Build history of the part. All positions in model axes, mm. A direction names the side the tool comes from. Give positions to 0.01 mm unless a question says otherwise; leave off trailing zeros. Loops run counter-clockwise (first coordinate to the right, second up) from the corner with the lowest first, then second, coordinate; pieces in that order, holes last. Notation, with made-up numbers: (9, -39.5) -> (61, -39.5) arc R18 cw to (61, -20.5) -> close; hole circle Ø11 at (66.25, 3.25). An arc over 180 degrees is marked (long way). Answer as a JSON object with one key per item and string values. Group by question number.
from build123d import *
from build123d.topology import SkipClean

# Parameters (mm, degrees)
SKETCH1_W           = 54
SKETCH1_H           = 28.5
SKETCH1_W_2         = 5
SKETCH1_H_2         = 22.5
SKETCH1_R           = 1.7
SKETCH1_R_2         = 7.5
BOSS_EXTRUDE2_DEPTH = 3
SKETCH2_W           = 4
SKETCH2_H           = 20.5
BOSS_EXTRUDE3_DEPTH = 21.75
SKETCH4_R           = 10.25
BOSS_EXTRUDE4_DEPTH = 4
SKETCH6_R           = 4.4
SKETCH6_R_2         = 1.45
CUT_EXTRUDE3_DEPTH  = 4
SKETCH7_R           = 1.45
CUT_EXTRUDE4_DEPTH  = 1.5
SKETCH8_W           = 28.781481152
SKETCH8_H           = 28.5
BOSS_EXTRUDE5_DEPTH = 3
SKETCH9_R           = 1.7
CUT_EXTRUDE5_DEPTH  = 3
SKETCH10_W          = 54
SKETCH10_H          = 28.5
SKETCH10_R          = 1.7
SKETCH10_W_2        = 5
SKETCH10_H_2        = 22.5
BOSS_EXTRUDE6_DEPTH = 15
SKETCH11_W          = 46
SKETCH11_H          = 15
CUT_EXTRUDE6_DEPTH  = 53.595151868


with BuildPart() as part:
    # Sketch1 → Boss-Extrude2 (new body)
    with BuildSketch(Plane(origin=(0, 0, 0), x_dir=(1, 0, 0), z_dir=(0, 1, 0))):
        Rectangle(SKETCH1_W, SKETCH1_H)
        with Locations((20.5, 0)):
            Rectangle(SKETCH1_W_2, SKETCH1_H_2, mode=Mode.SUBTRACT)
        with Locations((-20.5, 0)):
            Rectangle(SKETCH1_W_2, SKETCH1_H_2, mode=Mode.SUBTRACT)
        with Locations(Location((-9, -8.25, 0), (0, 0, 270))):
            Circle(SKETCH1_R, mode=Mode.SUBTRACT)
        with Locations(Location((9, -8.25, 0), (0, 0, 270))):
            Circle(SKETCH1_R, mode=Mode.SUBTRACT)
        with Locations(Location((-9, 8.25, 0), (0, 0, 270))):
            Circle(SKETCH1_R, mode=Mode.SUBTRACT)
        with Locations(Location((0, 0, 0), (0, 0, 270))):
            Circle(SKETCH1_R_2, mode=Mode.SUBTRACT)
        with Locations(Location((9, 8.25, 0), (0, 0, 270))):
            Circle(SKETCH1_R, mode=Mode.SUBTRACT)
    extrude(amount=BOSS_EXTRUDE2_DEPTH)

    # Sketch2 → Boss-Extrude3 (add)
    with BuildSketch(Plane(origin=(0, 3, 0), x_dir=(1, 0, 0), z_dir=(0, 1, 0))):
        with Locations((25, 0)):
            Rectangle(SKETCH2_W, SKETCH2_H)
    boss_extrude3 = extrude(amount=BOSS_EXTRUDE3_DEPTH)

    # Sketch4 → Boss-Extrude4 (add)
    with BuildSketch(Plane(origin=(27, 0, 0), x_dir=(0, 0, -1), z_dir=(1, 0, 0))):
        with Locations((0, 24.75)):
            Circle(SKETCH4_R)
    boss_extrude4 = extrude(amount=-BOSS_EXTRUDE4_DEPTH)

    # Mirror1: Boss-Extrude3, Boss-Extrude4 across plane
    add(boss_extrude3.mirror(Plane(origin=(0, 0, 0), x_dir=(0, 0, 1), z_dir=(1, 0, 0))))
    add(boss_extrude4.mirror(Plane(origin=(0, 0, 0), x_dir=(0, 0, 1), z_dir=(1, 0, 0))))

    # Sketch6 → Cut-Extrude3 (cut)
    with BuildSketch(Plane(origin=(27, 0, 0), x_dir=(0, 0, -1), z_dir=(1, 0, 0))):
        with Locations((0, 24.75)):
            Circle(SKETCH6_R)
        with Locations((0, 32.75)):
            Circle(SKETCH6_R_2)
        with Locations((8, 24.75)):
            Circle(SKETCH6_R_2)
        with Locations((0, 16.75)):
            Circle(SKETCH6_R_2)
        with Locations((-8, 24.75)):
            Circle(SKETCH6_R_2)
    cut_extrude3 = extrude(amount=-CUT_EXTRUDE3_DEPTH, mode=Mode.SUBTRACT)

    # Mirror3: Cut-Extrude3 across plane
    add(cut_extrude3.mirror(Plane(origin=(0, 0, 0), x_dir=(0, 0, 1), z_dir=(1, 0, 0))), mode=Mode.SUBTRACT)

    # Sketch7 → Cut-Extrude4 (cut)
    # profile 1 of 4: a face of its own
    with BuildSketch(Plane(origin=(27, 0, 0), x_dir=(0, 0, -1), z_dir=(1, 0, 0))):
        with BuildLine():
            ThreePointArc((10.25, 24.75), (10.200627247, 25.754840168), (10.052984631, 26.75))
            Line((10.052984631, 26.75), (8, 26.75))
            ThreePointArc((8, 26.75), (6, 24.75), (8, 22.75))
            Line((8, 22.75), (10.25, 22.75))
            Line((10.25, 22.75), (10.25, 24.75))
        make_face()
        with Locations((8, 24.75)):
            Circle(SKETCH7_R, mode=Mode.SUBTRACT)
    # profile 2 of 4: a face of its own
    with BuildSketch(Plane(origin=(27, 0, 0), x_dir=(0, 0, -1), z_dir=(1, 0, 0))):
        with BuildLine():
            Line((2, 32.75), (2, 34.802984631))
            ThreePointArc((2, 34.802984631), (0, 35), (-2, 34.802984631))
            Line((-2, 34.802984631), (-2, 32.75))
            ThreePointArc((-2, 32.75), (0, 30.75), (2, 32.75))
        make_face()
        with Locations((0, 32.75)):
            Circle(SKETCH7_R, mode=Mode.SUBTRACT)
    # profile 3 of 4: a face of its own
    with BuildSketch(Plane(origin=(27, 0, 0), x_dir=(0, 0, -1), z_dir=(1, 0, 0))):
        with BuildLine():
            Line((-8, 26.75), (-10.052984631, 26.75))
            ThreePointArc((-10.052984631, 26.75), (-10.200627247, 25.754840168), (-10.25, 24.75))
            Line((-10.25, 24.75), (-10.25, 22.75))
            Line((-10.25, 22.75), (-8, 22.75))
            ThreePointArc((-8, 22.75), (-6, 24.75), (-8, 26.75))
        make_face()
        with Locations((-8, 24.75)):
            Circle(SKETCH7_R, mode=Mode.SUBTRACT)
    # profile 4 of 4: a face of its own
    with BuildSketch(Plane(origin=(27, 0, 0), x_dir=(0, 0, -1), z_dir=(1, 0, 0))):
        with BuildLine():
            Line((-2, 16.75), (-2, 13.927640071))
            Line((-2, 13.927640071), (2, 13.927640071))
            Line((2, 13.927640071), (2, 16.75))
            ThreePointArc((2, 16.75), (0, 18.75), (-2, 16.75))
        make_face()
        with Locations((0, 16.75)):
            Circle(SKETCH7_R, mode=Mode.SUBTRACT)
    cut_extrude4 = extrude(amount=-CUT_EXTRUDE4_DEPTH, mode=Mode.SUBTRACT)

    # Mirror4: Cut-Extrude4 across plane
    add(cut_extrude4.mirror(Plane(origin=(0, 0, 0), x_dir=(0, 0, 1), z_dir=(1, 0, 0))), mode=Mode.SUBTRACT)

    # Sketch8 → Boss-Extrude5 (add)
    with BuildSketch(Plane(origin=(0, 3, 0), x_dir=(1, 0, 0), z_dir=(0, 1, 0))):
        Rectangle(SKETCH8_W, SKETCH8_H)
    extrude(amount=-BOSS_EXTRUDE5_DEPTH)

    # Sketch9 → Cut-Extrude5 (cut)
    with BuildSketch(Plane(origin=(0, 3, 0), x_dir=(1, 0, 0), z_dir=(0, 1, 0))):
        with BuildLine():
            ThreePointArc((-5.3, -7), (-5.797918472, -5.797918472), (-7, -5.3))
            Line((-7, -5.3), (-7, -7))
            Line((-7, -7), (-5.3, -7))
        make_face()
        with BuildLine():
            Line((-7, -7), (-7, -5.3))
            ThreePointArc((-7, -5.3), (-8.202081528, -8.202081528), (-5.3, -7))
            Line((-5.3, -7), (-7, -7))
        make_face()
        with BuildLine():
            ThreePointArc((8.7, -7), (8.202081528, -5.797918472), (7, -5.3))
            Line((7, -5.3), (7, -7))
            Line((7, -7), (5.3, -7))
            ThreePointArc((5.3, -7), (7, -8.7), (8.7, -7))
        make_face()
        with BuildLine():
            Line((7, -7), (7, -5.3))
            ThreePointArc((7, -5.3), (5.797918472, -5.797918472), (5.3, -7))
            Line((5.3, -7), (7, -7))
        make_face()
        with BuildLine():
            ThreePointArc((8.7, 7), (7, 8.7), (5.3, 7))
            Line((5.3, 7), (7, 7))
            Line((7, 7), (7, 5.3))
            ThreePointArc((7, 5.3), (8.202081528, 5.797918472), (8.7, 7))
        make_face()
        with BuildLine():
            Line((7, 7), (5.3, 7))
            ThreePointArc((5.3, 7), (5.797918472, 5.797918472), (7, 5.3))
            Line((7, 5.3), (7, 7))
        make_face()
        with Locations(Location((-7, 7, 0), (0, 0, 270))):
            Circle(SKETCH9_R)
    extrude(amount=-CUT_EXTRUDE5_DEPTH, mode=Mode.SUBTRACT)

    # Sketch10 → Boss-Extrude6 (add)
    with SkipClean():  # the faces are left unmerged after this step: merging them gives an invalid solid
        with BuildSketch(Plane.XZ):
            Rectangle(SKETCH10_W, SKETCH10_H)
            with Locations(Location((-7, 7, 0), (0, 0, 90))):
                Circle(SKETCH10_R, mode=Mode.SUBTRACT)
            with Locations(Location((-7, -7, 0), (0, 0, 90))):
                Circle(SKETCH10_R, mode=Mode.SUBTRACT)
            with Locations(Location((7, -7, 0), (0, 0, 90))):
                Circle(SKETCH10_R, mode=Mode.SUBTRACT)
            with Locations(Location((7, 7, 0), (0, 0, 90))):
                Circle(SKETCH10_R, mode=Mode.SUBTRACT)
            with Locations((-20.5, 0)):
                Rectangle(SKETCH10_W_2, SKETCH10_H_2, mode=Mode.SUBTRACT)
            with Locations((20.5, 0)):
                Rectangle(SKETCH10_W_2, SKETCH10_H_2, mode=Mode.SUBTRACT)
        extrude(amount=BOSS_EXTRUDE6_DEPTH)

    # Sketch11 → Cut-Extrude6 (cut, through all)
    with BuildSketch(Plane.XY.offset(14.25)):
        with Locations((0, -4.5)):
            Rectangle(SKETCH11_W, SKETCH11_H)
    extrude(amount=-CUT_EXTRUDE6_DEPTH, mode=Mode.SUBTRACT)


solid = part.part
(1) Saw through at B-B on y = 5.5. List the corners of the cut face in (x, z).
(2) Saw through at D-D on z = -12. List the corners of the cut face in (x, y).
(3) Pull direction X, two halves, no side cores. Call faces 1 (the flat face through (-26, 15, -2)), 2 (the flat face through (20, -13, -11.25)), 3 (the flat face through (-25.5, 25, -10)): pulls with the +X half, pulls with the -X half, needs draft (parallel to the pull), parting line crosses it, or undercut.
(4) Saw through at A-A on x = -19. List the corners of the cut face in (y, z), plus the area to 3 significant figures.
(5) Pin check, flat tips, straight feed: pin 1 (0.8 mm diameter, centred on x = -26, y = 16, fed in from -Z); pin 2 (4.5 mm diameter, centred on y = 24.5, z = 8, fed in from -X); pin 3 (1.6 mm diameter, centred on x = 26.5, y = 33.5, fed in from +Z); pin 4 (1.2 mm diameter, centred on x = -26.5, z = -9.5, fed in from +Y). Stop position of each tip, or through.
(6) Probe line 1 along Y through (x, z) = (-24.15, 0); line 2 along X through (y, z) = (-12.65, 7); line 3 along X through (y, z) = (-6.5, -11.25). List the from-to ranges inside material, lowest first. Write a range as [from, to].
(7) Saw through at C-C on x = 7. List the corners of the cut face in (y, z).
(8) 3-axis set-ups, long thin cutter, end or side, ignore diameter. For faces 4 (the flat face through (25, 14, -10.25)), 5 (the flat face through (-25, 3, 12)), 6 (the cylindrical face through (-26.3, 24.7, 6)), 7 (the cylindrical face through (26.3, 24.7, 6)): which of +Z, -Z, +X, -X, +Y, -Y reach the whole face in a straight line?
Calculated:
{
 "1": {"outline": "(-27, -10.25) -> (-23, -10.25) -> (-23, 10.25) -> (-27, 10.25) -> close; (23, -10.25) -> (27, -10.25) -> (27, 10.25) -> (23, 10.25) -> close"},
 "2": {"outline": "(-27, -15) -> (27, -15) -> (27, 3) -> (23, 3) -> (23, -12) -> (-23, -12) -> (-23, 3) -> (-27, 3) -> close"},
 "3": {"face 1": "needs draft", "face 2": "undercut", "face 3": "pulls with the -X half"},
 "4": {"outline": "(-15, -14.25) -> (-12, -14.25) -> (-12, -11.25) -> (-15, -11.25) -> close; (-15, 11.25) -> (-12, 11.25) -> (-12, 14.25) -> (-15, 14.25) -> close", "area": "18.0 mm^2"},
 "5": {"pin 1": "stops at z = -10.25", "pin 2": "stops at x = -27", "pin 3": "stops at z = 6.47", "pin 4": "stops at y = 29.83"},
 "6": {"line 1": "y = [-15, 15.3], [18.2, 20.35], [29.15, 31.3], [34.2, 35]", "line 2": "x = [-27, -23], [-18, -8.7], [-5.3, 5.3], [8.7, 18], [23, 27]", "line 3": "x = [-27, -23], [23, 27]"},
 "7": {"outline": "(-15, -14.25) -> (-12, -14.25) -> (-12, -8.7) -> (-15, -8.7) -> close; (-15, -5.3) -> (-12, -5.3) -> (-12, 5.3) -> (-15, 5.3) -> close; (-15, 8.7) -> (-12, 8.7) -> (-12, 14.25) -> (-15, 14.25) -> close"},
 "8": {"face 4": "-Z, +X, -X, +Y", "face 5": "+Z, +X, -X, +Y", "face 6": "+Z, -X", "face 7": "+Z, +X"}
}
